from build123d import *

# Parameters (mm, degrees)
F1_DEPTH       = 14
F3_DEPTH       = 5
F5_D           = 10
F6_R           = 8
F7_DEPTH       = 4
F9_D           = 6.6
F9_CBORE_D     = 11.25
F9_CBORE_DEPTH = 6
F11_D          = 3.2
F11_DEPTH      = 9
F11_TIP        = 0.9613769904


with BuildPart() as f1:
    # F0 (on Top) → F1 (new body)
    with BuildSketch(Plane.XY):
        with BuildLine():
            Line((8.4736176887, -30), (70, -30))
            Line((70, -30), (70, 30))
            Line((70, 30), (-70, 30))
            Line((-70, 30), (-70, -30))
            Line((-70, -30), (-8.4949249349, -30))
            Line((-8.4949249349, -30), (-8.4949249349, -10.2936840984))
            ThreePointArc((-8.4949249349, -10.2936840984), (-8.5, -10), (-8.4949249349, -9.7063159016))
            ThreePointArc((-8.4949249349, -9.7063159016), (0.4815504321, -1.5136515991), (8.4736176887, -10.6691810406))
            Line((8.4736176887, -10.6691810406), (8.4736176887, -30))
        make_face()
    extrude(amount=F1_DEPTH)

    # F2 (on face) → F3 (cut)
    with BuildSketch(Plane.XY.offset(14)):
        with BuildLine():
            Line((12.9707033085, -30), (12.9707033085, -10.8722704179))
            Line((12.9707033085, -10.8722704179), (12.9707033085, -9.1277295821))
            ThreePointArc((12.9707033085, -9.1277295821), (0.3687690423, 2.9947685394), (-12.900361613, -8.3935535324))
            Line((-12.900361613, -8.3935535324), (-12.900361613, -11.6064464676))
            Line((-12.900361613, -11.6064464676), (-12.900361613, -30))
            Line((-12.900361613, -30), (-8.4949249349, -30))
            Line((-8.4949249349, -30), (-8.4949249349, -10.2936840984))
            ThreePointArc((-8.4949249349, -10.2936840984), (0.1880504934, -1.5020804304), (8.4736176887, -10.6691810406))
            Line((8.4736176887, -10.6691810406), (8.4736176887, -30))
            Line((8.4736176887, -30), (12.9707033085, -30))
        make_face()
    extrude(amount=-F3_DEPTH, mode=Mode.SUBTRACT)

    # F5 (through all)
    with Locations(Plane.XY.offset(14)):
        with Locations((-30, 18)):
            Hole(F5_D / 2)

    # F6 (on face) → F7 (cut)
    with BuildSketch(Plane(origin=(0, 0, 0), x_dir=(1, 0, 0), z_dir=(0, 0, -1))):
        with Locations((-55, 10.2936840984)):
            Circle(F6_R)
        with Locations((55, 10.2936840984)):
            Circle(F6_R)
    extrude(amount=-F7_DEPTH, mode=Mode.SUBTRACT)

    # F9 (through all)
    with Locations(Plane.XY.offset(14)):
        with Locations((-55, -10), (55, -10)):
            CounterBoreHole(F9_D / 2, F9_CBORE_D / 2, F9_CBORE_DEPTH)

    # F11
    with Locations(Plane(origin=(0, 30, 0), x_dir=(-1, 0, 0), z_dir=(0, 1, 0))):
        with Locations((30, 7)):
            Hole(F11_D / 2, depth=F11_DEPTH)
            with Locations((0, 0, -(F11_DEPTH + F11_TIP / 2))):  # 118° drill point
                Cone(0, F11_D / 2, F11_TIP, mode=Mode.SUBTRACT)


solid = f1.part
Can you work these out from the model? Positions are in its coordinate system, mm. A direction names the side the tool comes from. Round coordinates to 2 decimals unless told otherwise and drop trailing zeros. Write each loop counter-clockwise with the first axis right and the second up, starting at its lowest first coordinate (ties: lowest second). Pieces come first, ordered by that corner, then holes. Notation, with made-up numbers: M -17,-40 L -3,-40 A26 ccw -3,-26 Z; hole C 27,30 d7. An arc over 180 degrees is marked long. Use a Markdown table: item, result.
Item 1: I want a section at A-A (x = 55). List the corners of the cut face in (y, z) for me (3 decimals), and give its area (3 significant figures).
Found:
| item | result |
|---|---|
| outline | M -30,0 L -18.294,0 L -18.294,4 L -13.3,4 L -13.3,8 L -15.625,8 L -15.625,14 L -30,14 Z; M -6.7,4 L -2.294,4 L -2.294,0 L 30,0 L 30,14 L -4.375,14 L -4.375,8 L -6.7,8 Z |
| area | 682 mm2 |
Item 2: We'd pull the mould along Y, two halves only. Please class faces 1 (the face through (-49.8, -12.15, 11.04)), 2 (the face through (-1, 7, 14)), 3 (the face through (-40, -30, 7)): released by +Y, released by -Y, zero draft, split by the parting line, or undercut.
Found:
| item | result |
|---|---|
| face 1 | undercut |
| face 2 | zero draft |
| face 3 | released by -Y |
Item 3: If I drill on line 1 along Z through (x, y) = (-30, 25.75); line 2 along Y through (x, z) = (55, 7.25); line 3 along X through (y, z) = (-11.5, 9.5), over which ranges is the centre line in solid material (lowest first)? Write a range as [from, to].
Found:
| item | result |
|---|---|
| line 1 | z = [0, 5.4], [8.6, 14] |
| line 2 | y = [-30, -13.3], [-6.7, 30] |
| line 3 | x = [-70, -60.42], [-49.58, -12.9], [12.97, 49.58], [60.42, 70] |
Item 4: For pin 1 Ø5.5 at (x, y) = (-55, -9) entering from +Z; pin 2 Ø5 at (x, y) = (-58.5, -6.5) entering from -Z; pin 3 Ø5.5 at (x, y) = (-55, -10) entering from +Z; pin 4 Ø3 at (x, z) = (-30, 7) entering from +Y, each with a flat end and sliding along its axis, tell me the tip position at first contact or that it passes through.
Found:
| item | result |
|---|---|
| pin 1 | stops at z = 8 |
| pin 2 | stops at z = 4 |
| pin 3 | passes through |
| pin 4 | stops at y = 13.23 |
Item 5: I want a section at D-D (y = 18). List the corners of the cut face in (x, z) for me, and give its area (3 significant figures).
Found:
| item | result |
|---|---|
| outline | M -70,0 L -35,0 L -35,14 L -70,14 Z; M -25,0 L 70,0 L 70,14 L -25,14 Z |
| area | 1,820 mm2 |
Item 6: I want a section at C-C (z = 11). List the corners of the cut face in (x, y) for me (3 decimals).
Found:
| item | result |
|---|---|
| outline | M -70,-30 L -12.9,-30 L -12.9,-8.394 A13 cw 12.971,-9.128 L 12.971,-30 L 70,-30 L 70,30 L -70,30 Z; hole C -55,-10 d11.25; hole C -30,18 d10; hole C 55,-10 d11.25 |
Item 7: I want a section at B-B (y = -22). List the corners of the cut face in (x, z) for me.
Found:
| item | result |
|---|---|
| outline | M -70,0 L -8.49,0 L -8.49,9 L -12.9,9 L -12.9,14 L -70,14 Z; M 8.47,0 L 70,0 L 70,14 L 12.97,14 L 12.97,9 L 8.47,9 Z |
Item 8: Which directions (+Z, -Z, +X, -X, +Y, -Y) give clear straight access to the entire face, cutting with the end or side of a thin tool? Please do faces 4 (the face through (-9, -13, 9)), 5 (the face through (-31.27, 26.31, 6.03)), 6 (the face through (59, -10, 8)), 7 (the face through (58.44, -10.41, 4)), 8 (the face through (8.474, -20, 4)).
Found:
| item | result |
|---|---|
| face 4 | +Z, -Y |
| face 5 | +Y |
| face 6 | +Z |
| face 7 | -Z |
| face 8 | +Z, -Z, -Y |
